```python
from build123d import *

# Parameters (mm, degrees)
ALUM_C_CHNL_LONGBOSS_EXTRUDE2_DEPTH      = 305.8
ALUM_C_CHNL_LONGBOSS_EXTRUDE2_DEPTH_BACK = 305.8
FILLET1_R                                = 10
SKETCH7_R                                = 3.25
CUT_EXTRUDE4_DEPTH                       = 20
LPATTERN2_COUNT                          = 30
LPATTERN2_PITCH                          = 10
LPATTERN1_COUNT                          = 30
LPATTERN1_PITCH                          = 10
SKETCH10_R                               = 3.25
CUT_EXTRUDE8_DEPTH                       = 3.175


with BuildPart() as part:
    # Sketch2 → Alum C chnl LONGBoss-Extrude2 (new body, two sides)
    with BuildSketch(Plane.XY) as alum_c_chnl_longboss_extrude2_sk:
        Polygon((-304.8, 12.7), (-304.8, 15.875), (-257.175, 15.875), (-257.175, 111.125), (-304.8, 111.125), (-304.8, 114.3), (-254, 114.3), (-254, 12.7), align=None)
    extrude(amount=ALUM_C_CHNL_LONGBOSS_EXTRUDE2_DEPTH)
    extrude(alum_c_chnl_longboss_extrude2_sk.sketch, amount=-ALUM_C_CHNL_LONGBOSS_EXTRUDE2_DEPTH_BACK)

    # Fillet1
    fillet1_edges = [part.edges().sort_by_distance(p)[0] for p in [
        (-304.8, 112.7125, -305.8),
        (-304.8, 112.7125, 305.8),
        (-304.8, 14.2875, 305.8),
        (-304.8, 14.2875, -305.8),
    ]]
    fillet(fillet1_edges, radius=FILLET1_R)

    # Sketch7 → Cut-Extrude4 (cut)
    with BuildSketch(Plane(origin=(0, 114.3, 0), x_dir=(1, 0, 0), z_dir=(0, 1, 0))):
        with Locations((-280.2, 0)):
            Circle(SKETCH7_R)
    cut_extrude4 = extrude(amount=-CUT_EXTRUDE4_DEPTH, mode=Mode.SUBTRACT)

    # LPattern2: Cut-Extrude4 ×30
    with Locations(*[(0, 0, -i * LPATTERN2_PITCH) for i in range(1, LPATTERN2_COUNT)]):
        add(cut_extrude4, mode=Mode.SUBTRACT)

    # LPattern1: Cut-Extrude4 ×30
    with Locations(*[(0, 0, i * LPATTERN1_PITCH) for i in range(1, LPATTERN1_COUNT)]):
        add(cut_extrude4, mode=Mode.SUBTRACT)

    # Sketch10 → Cut-Extrude8 (cut)
    with BuildSketch(Plane(origin=(0, 15.875, 0), x_dir=(1, 0, 0), z_dir=(0, 1, 0))):
        with Locations((-285, 275)):
            Circle(SKETCH10_R)
        with Locations((-285, 0)):
            Circle(SKETCH10_R)
        with Locations((-285, -275)):
            Circle(SKETCH10_R)
    extrude(amount=-CUT_EXTRUDE8_DEPTH, mode=Mode.SUBTRACT)


solid = part.part
```
Check sheet for the modelled part. Datum: model origin and axes. Units: mm. A direction names the side the tool comes from. Give positions to 0.01 mm unless a question says otherwise; leave off trailing zeros. Write each loop counter-clockwise with the first axis right and the second up, starting at its lowest first coordinate (ties: lowest second). Pieces come first, ordered by that corner, then holes. Notation, with made-up numbers: (43.25, 87) - (100.25, 87) arc R27 ccw to (100.25, 103) - close; hole circle Ø7 at (51.25, 52). An arc over 180 degrees is marked (long way). Answer as a JSON object with one key per item and string values. Group by question number.
1) Release check for a two-part mould opening along Y. For faces 3 (the face through (-281, 15.875, 4)), 4 (the face through (-280, 114.3, 4)), 5 (the face through (-279, 12.7, 4)), 6 (the face through (-256, 64, -305.8)) record: pulls with the +Y half, pulls with the -Y half, needs draft (parallel to the pull), parting line crosses it, or undercut.
2) Access from +Z, -Z, +X, -X, +Y, -Y to the whole of each face (thin tool, end or side, straight path). Record for faces 1 (the face through (-257.175, 63, 4)), 2 (the face through (-301.95, 112.73, -302.79)).
3) Depth check by flat-ended pin: P1, Ø6, axis at x = -280.2, z = -290, coming from the +Y side (3 decimals). Enter the tip coordinate at first touch or a pass-through.
4) Thickness scan on probe 1 along Y at (x, z) = (-281.5, 65) (3 decimals); probe 2 along X at (y, z) = (112.3, 70); probe 3 along X at (y, z) = (54, 148) (3 decimals). Record the ranges inside material, lowest first. Write a range as from..to.
5) Sectioned sample at A-A (y = 21.5). Record the cut outline in (x, z) (3 decimals), then the cut area to 3 significant figures.
Geometry results:
{
 "1": {"face 3": "undercut", "face 4": "pulls with the +Y half", "face 5": "pulls with the -Y half", "face 6": "needs draft"},
 "2": {"face 1": "+Z, -Z, -X", "face 2": "-Z, -X, +Y, -Y"},
 "3": {"P1": "stops at y = 15.875"},
 "4": {"probe 1": "y = 12.7..15.875, 111.125..114.3", "probe 2": "x = -304.8..-283.45, -276.95..-254", "probe 3": "x = -257.175..-254"},
 "5": {"outline": "(-257.175, -305.8) - (-254, -305.8) - (-254, 305.8) - (-257.175, 305.8) - close", "area": "1,940 mm^2"}
}
